```python
from build123d import *

# Parameters (mm, degrees)
BASPROSKE_W         = 15
BASPROSKE_H         = 18
TOOTHCUT_DEPTH      = 30.546573405
TEETHCUTS_COUNT     = 16
TEETHCUTS_ANGLE     = 337.5
HUBNEABOTSKE_R      = 5
HUBNEARBOTH_DEPTH   = 15.0000254
HUBFAR_START        = 15.0000254
HUBFARSKE_R         = 5
HUBFAR_DEPTH        = 15.0000254
BORSKE_R            = 2.5
BORE_DEPTH          = 45.0000508
CUT_EXTRUDE1_START  = -15.0000254
SKETCH3_R           = 5
CUT_EXTRUDE1_DEPTH  = 15.0000254
BOSS_EXTRUDE1_START = -20
SKETCH5_R           = 2.5
BOSS_EXTRUDE1_DEPTH = 20
BOSS_EXTRUDE2_START = 1
SKETCH6_R           = 7.5
SKETCH6_R_2         = 5
BOSS_EXTRUDE2_DEPTH = 1
SKETCH7_R           = 7.5
SKETCH7_R_2         = 3.4375
CUT_EXTRUDE2_DEPTH  = 30.757152718
BOSS_EXTRUDE3_START = 10.0000254
SKETCH8_R           = 2.5
BOSS_EXTRUDE3_DEPTH = 10.0000254
SKETCH10_OUTSIDE_W  = 49.174
SKETCH10_OUTSIDE_H  = 49.174
SKETCH10_OUTSIDE_R  = 3.4375
CUT_EXTRUDE3_DEPTH  = 14.0000254
CUT_EXTRUDE4_START  = -8
SKETCH12_R          = 3.4375
CUT_EXTRUDE4_DEPTH  = 8


with BuildPart() as part:
    # BasProSke → Base-Revolve (revolve)
    with BuildSketch(Plane(origin=(0, 0, 0), x_dir=(1, 0, 0), z_dir=(0, 1, 0)), mode=Mode.PRIVATE) as base_revolve_sk:
        with Locations((7.5, 9)):
            Rectangle(BASPROSKE_W, BASPROSKE_H)
    revolve(base_revolve_sk.sketch.rotate(Axis((-10, 0, 0), (1, 0, 0)), 180), axis=Axis((-10, 0, 0), (1, 0, 0)))

    # TooCutSke → ToothCut (cut, through all)
    with BuildSketch(Plane(origin=(0, 0, 0), x_dir=(0, 0, -1), z_dir=(1, 0, 0))):
        with BuildLine():
            ThreePointArc((1.03434411, 13.459313997), (0, 13.499), (-1.03434411, 13.459313997))
            ThreePointArc((-1.03434411, 13.459313997), (-1.635143665, 15.806872195), (-3.065655864, 17.762792553))
            ThreePointArc((-3.065655864, 17.762792553), (0, 18.0254), (3.065655864, 17.762792553))
            ThreePointArc((3.065655864, 17.762792553), (1.635143665, 15.806872195), (1.03434411, 13.459313997))
        make_face()
    toothcut = extrude(amount=TOOTHCUT_DEPTH, mode=Mode.SUBTRACT)

    # TeethCuts: ToothCut ×16 about axis
    teethcuts_axis = Axis((-10, 0, 0), (1, 0, 0))
    for i in range(1, TEETHCUTS_COUNT):
        add(toothcut.rotate(teethcuts_axis, i * TEETHCUTS_ANGLE / (TEETHCUTS_COUNT - 1)), mode=Mode.SUBTRACT)

    # HubNeaBotSke → HubNearBoth (add)
    with BuildSketch(Plane.ZY):
        with Locations(Location((0, 0, 0), (0, 0, 180))):
            Circle(HUBNEABOTSKE_R)
    extrude(amount=HUBNEARBOTH_DEPTH)

    # HubFarSke → HubFar (add)
    with BuildSketch(Plane(origin=(15, 0, 0), x_dir=(0, 0, -1), z_dir=(1, 0, 0)).offset(HUBFAR_START)):
        Circle(HUBFARSKE_R)
    extrude(amount=-HUBFAR_DEPTH)

    # BorSke → Bore (cut, symmetric)
    with BuildSketch(Plane(origin=(0, 0, 0), x_dir=(0, 0, -1), z_dir=(1, 0, 0))):
        with Locations(Location((0, 0, 0), (0, 0, 180))):
            Circle(BORSKE_R)
    extrude(amount=BORE_DEPTH, both=True, mode=Mode.SUBTRACT)

    # Sketch3 → Cut-Extrude1 (cut)
    with BuildSketch(Plane.ZY.offset(15.0000254).offset(CUT_EXTRUDE1_START)):
        Circle(SKETCH3_R)
    extrude(amount=CUT_EXTRUDE1_DEPTH, mode=Mode.SUBTRACT)

    # Sketch5 → Boss-Extrude1 (add)
    with BuildSketch(Plane.ZY.offset(BOSS_EXTRUDE1_START)):
        Circle(SKETCH5_R)
    extrude(amount=BOSS_EXTRUDE1_DEPTH)

    # Sketch6 → Boss-Extrude2 (add)
    with BuildSketch(Plane(origin=(15, 0, 0), x_dir=(0, 0, -1), z_dir=(1, 0, 0)).offset(BOSS_EXTRUDE2_START)):
        with Locations(Location((0, 0, 0), (0, 0, 180))):
            Circle(SKETCH6_R)
        Circle(SKETCH6_R_2, mode=Mode.SUBTRACT)
    extrude(amount=-BOSS_EXTRUDE2_DEPTH)

    # Sketch7 → Cut-Extrude2 (cut, through all)
    with BuildSketch(Plane(origin=(16, 0, 0), x_dir=(0, 0, -1), z_dir=(1, 0, 0))):
        with Locations(Location((0, 0, 0), (0, 0, 180))):
            Circle(SKETCH7_R)
        Circle(SKETCH7_R_2, mode=Mode.SUBTRACT)
    extrude(amount=CUT_EXTRUDE2_DEPTH, mode=Mode.SUBTRACT)

    # Sketch8 → Boss-Extrude3 (add)
    with BuildSketch(Plane(origin=(20, 0, 0), x_dir=(0, 0, -1), z_dir=(1, 0, 0)).offset(BOSS_EXTRUDE3_START)):
        Circle(SKETCH8_R)
    extrude(amount=-BOSS_EXTRUDE3_DEPTH)

    # Sketch10 outside → Cut-Extrude3 (cut)
    # profile 1 of 2: a face of its own
    with BuildSketch(Plane(origin=(30.0000254, 0, 0), x_dir=(0, 0, -1), z_dir=(1, 0, 0))):
        Rectangle(SKETCH10_OUTSIDE_W, SKETCH10_OUTSIDE_H)
        Circle(SKETCH10_OUTSIDE_R, mode=Mode.SUBTRACT)
    # profile 2 of 2: a face of its own
    with BuildSketch(Plane(origin=(30.0000254, 0, 0), x_dir=(0, 0, -1), z_dir=(1, 0, 0))):
        with BuildLine():
            Line((-2.050495367, 1.925), (2.050495367, 1.925))
            ThreePointArc((2.050495367, 1.925), (2.8125, 0), (2.050495367, -1.925))
            Line((2.050495367, -1.925), (-2.050495367, -1.925))
            ThreePointArc((-2.050495367, -1.925), (-2.8125, 0), (-2.050495367, 1.925))
        make_face()
    extrude(amount=-CUT_EXTRUDE3_DEPTH, mode=Mode.SUBTRACT)

    # Sketch12 → Cut-Extrude4 (cut)
    with BuildSketch(Plane(origin=(30.0000254, 0, 0), x_dir=(0, 0, -1), z_dir=(1, 0, 0)).offset(CUT_EXTRUDE4_START)):
        Circle(SKETCH12_R)
    extrude(amount=CUT_EXTRUDE4_DEPTH, mode=Mode.SUBTRACT)


solid = part.part
```
The listing builds one solid part. Answer for the finished solid, in the listing's coordinates (mm). A direction names the side the tool comes from. Give positions to 0.01 mm unless a question says otherwise; leave off trailing zeros. Order: outer loops, then holes, each group sorted by start corner. A loop starts at its lowest first (then second) coordinate and runs counter-clockwise, first axis right, second up. Notation, with made-up numbers: (-8, -16) - (7, -16) arc R8 ccw to (7, -4) - close; hole circle Ø11 at (86, 5). An arc over 180 degrees is marked (long way). Answer in a Markdown table with one row per item. Add a question column.
Q1. The part is cut by section C-C (z = -7). Determine the outline of the cut face in (x, y).
Q2. Find the intervals of material crossed by line 1 along Z through (x, y) = (7, 9); line 2 along Y through (x, z) = (7.5, -13); line 3 along Y through (x, z) = (8.5, 15), in increasing order. Write a range as [from, to].
Q3. Which of the six approach directions +Z, -Z, +X, -X, +Y, -Y give full straight-line access (tool end or side, diameter ignored) to faces 1 (the cylindrical face through (7.4, 1.64, 15.82)), 2 (the cylindrical face through (7.4, -15.82, 1.64)), 3 (the cylindrical face through (7.4, -12.48, -5.15)), 4 (the cylindrical face through (7.395, 15.762, 1.614))?
Q4. The part is cut by section A-A (y = 0). Determine the outline of the cut face in (x, z), then the cut area to 3 significant figures.
Q5. The part is cut by section B-B (z = 0). Determine the outline of the cut face in (x, y) (1 decimal), then the cut area to 3 significant figures.
Q6. Given P1, Ø1.5, axis at y = 9.5, z = -11.5, coming from the +X side; P2, Ø4, axis at x = 9, y = 0.5, coming from the -Z side; P3, Ø8, axis at x = 4.5, y = -1.5, coming from the +Z side; P4, Ø5, axis at x = 11, z = 0.5, coming from the -Y side, each flat-ended and moving along its own axis, determine where each tip first touches the part or whether it passes through.
Q7. For a pull along Z with two mould halves and no side action, classify faces 5 (the cylindrical face through (7.605, 17.655, 3.505)), 6 (the cylindrical face through (7.4, 0, -13.5)), 7 (the cylindrical face through (7.4, -4.54, -15.18)) as released by +Z, released by -Z, zero draft, split by the parting line, or undercut.
Determined:
| question | item | result |
|---|---|---|
| 1 | outline | (0, -13.4) - (15, -13.4) - (15, -2.69) - (16, -2.69) - (16, 2.69) - (15, 2.69) - (15, 13.4) - (0, 13.4) - close |
| 2 | line 1 | z = [-14.96, -10.5], [-10.06, 10.06], [10.5, 14.96] |
| 2 | line 2 | y = [-10.22, -6.68], [-4.25, 4.25], [6.68, 10.22] |
| 2 | line 3 | y = [-9.95, -9.07], [-4.55, -1.32], [1.32, 4.55], [9.07, 9.95] |
| 3 | face 1 | +Z, +X, -X |
| 3 | face 2 | +X, -X, -Y |
| 3 | face 3 | +X, -X |
| 3 | face 4 | +X, -X, +Y |
| 4 | outline | (0, -13.5) - (15, -13.5) - (15, -7.5) - (16, -7.5) - (16, -3.44) - (22, -3.44) - (22, -2.81) - (16, -2.81) - (16, 2.81) - (22, 2.81) - (22, 3.44) - (16, 3.44) - (16, 7.5) - (15, 7.5) - (15, 13.5) - (0, 13.5) - close |
| 4 | area | 427 mm² |
| 5 | outline | (0, -13.5) - (15, -13.5) - (15, -7.5) - (16, -7.5) - (16, -3.4) - (22, -3.4) - (22, -1.9) - (16, -1.9) - (16, 1.9) - (22, 1.9) - (22, 3.4) - (16, 3.4) - (16, 7.5) - (15, 7.5) - (15, 13.5) - (0, 13.5) - close |
| 5 | area | 438 mm² |
| 6 | P1 | stops at x = 15 |
| 6 | P2 | stops at z = -17.16 |
| 6 | P3 | stops at z = 17.74 |
| 6 | P4 | stops at y = -17.7 |
| 7 | face 5 | released by +Z |
| 7 | face 6 | released by -Z |
| 7 | face 7 | undercut |
